Build history of the part. All positions in model axes, mm. Coordinates: 2 decimals unless noted, no trailing zeros. Order: outer loops, then holes, each group sorted by start corner. A loop starts at its lowest first (then second) coordinate and runs counter-clockwise, first axis right, second up. Notation, with made-up numbers: (36, 43) - (69, 43) arc R32 ccw to (69, 74) - close; hole circle Ø5 at (-14, 26.25). An arc over 180 degrees is marked (long way). Return JSON: item names as keys, results as strings.
from build123d import *

# Parameters (mm, degrees)
SKETCH2_R   = 3.175
SKETCH2_R_2 = 2.286


with BuildPart() as part:
    # Sweep1: sweep along a path in Sketch1
    with BuildLine(Plane.XY) as sweep1_path:
        Line((-15.200789542, -14.78287466), (5.094778342, -14.78287466))
        ThreePointArc((5.094778342, -14.78287466), (10.025281152, -15.431987669), (14.619778342, -17.335090718))
        Line((14.619778342, -17.335090718), (38.774210458, -31.280658602))
        ThreePointArc((38.774210458, -31.280658602), (43.368707649, -33.183761651), (48.299210458, -33.83287466))
        Line((48.299210458, -33.83287466), (444.490346227, -33.83287466))
        ThreePointArc((444.490346227, -33.83287466), (449.420849036, -33.183761651), (454.015346227, -31.280658602))
        Line((454.015346227, -31.280658602), (483.669039656, -14.160090718))
        ThreePointArc((483.669039656, -14.160090718), (488.263536847, -12.256987669), (493.194039656, -11.60787466))
        Line((493.194039656, -11.60787466), (526.189607541, -11.60787466))
    # Sketch2 → Sweep1 (sweep)
    with BuildSketch(Plane(origin=(-15.200789542, -14.78287466, 0), x_dir=(0, 0, -1), z_dir=(1, 0, 0))):
        Circle(SKETCH2_R)
        Circle(SKETCH2_R_2, mode=Mode.SUBTRACT)
    sweep(path=sweep1_path.line)


solid = part.part
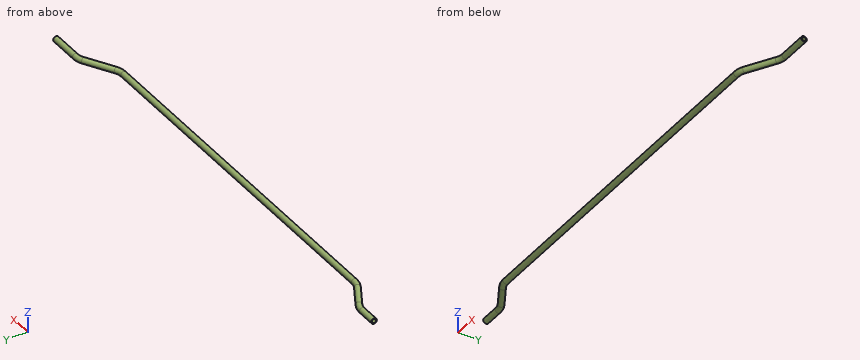
1. Drop flat-ended pins along their axis: pin 1 (3 mm diameter, centred on y = -27.5, z = 0.5, fed in from -X); pin 2 (10 mm diameter, centred on x = 342, y = -26, fed in from +Z); pin 3 (2 mm diameter, centred on x = 116.5, z = 1, fed in from +Y). Give the stop position or say it passes through.
Check values:
{"pin 1": "x = 23.33", "pin 2": "z = 1.43", "pin 3": "y = -30.66"}
2. Cut at A-A on x = 141. Give the cut face in (y, z) (3 decimals).
Check values:
{"outline": "circle Ø6.35 at (-33.833, 0); hole circle Ø4.572 at (-33.833, 0)"}
3. Probe L1, parallel to Y at x = -10.5, z = 0; L2, parallel to Y at x = 253.5, z = 0; L3, parallel to X at y = -22.25, z = 1. List the from-to ranges inside material, lowest first.
Check values:
{"L1": "-17.96 to -17.07, -12.5 to -11.61", "L2": "-37.01 to -36.12, -31.55 to -30.66", "L3": "17.11 to 19.02, 27.24 to 29.16, 463.63 to 465.55, 473.77 to 475.68"}
